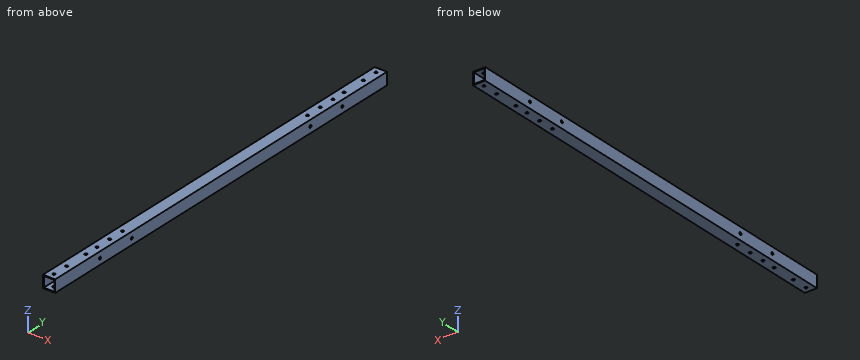
```python
from build123d import *

# Parameters (mm, degrees)
SKETCH_1_W          = 15
SKETCH_1_H          = 15
SKETCH_1_W_2        = 13
SKETCH_1_H_2        = 13
EXTRUDE_1_DEPTH     = 520
SKETCH_2_R          = 1.6
CUT_EXTRUDE_1_DEPTH = 521.270362408
SKETCH_3_R          = 1.6
CUT_EXTRUDE_2_DEPTH = 521.270362408


with BuildPart() as part:
    # 草图1 → 拉伸-薄壁1 (new body)
    with BuildSketch(Plane(origin=(0, 0, 0), x_dir=(1, 0, 0), z_dir=(0, 1, 0))):
        Rectangle(SKETCH_1_W, SKETCH_1_H)
        Rectangle(SKETCH_1_W_2, SKETCH_1_H_2, mode=Mode.SUBTRACT)
    extrude(amount=EXTRUDE_1_DEPTH)

    # 草图2 → 切除-拉伸1 (cut, through all)
    with BuildSketch(Plane.XY.offset(7.5)):
        with Locations((0, 7.5)):
            Circle(SKETCH_2_R)
        with Locations((0, 27.5)):
            Circle(SKETCH_2_R)
        with Locations((0, 57.5)):
            Circle(SKETCH_2_R)
        with Locations((0, 75)):
            Circle(SKETCH_2_R)
        with Locations((0, 95)):
            Circle(SKETCH_2_R)
        with Locations((0, 115)):
            Circle(SKETCH_2_R)
        with Locations(Location((0, 405, 0), (0, 0, 180))):
            Circle(SKETCH_2_R)
        with Locations(Location((0, 425, 0), (0, 0, 180))):
            Circle(SKETCH_2_R)
        with Locations(Location((0, 445, 0), (0, 0, 180))):
            Circle(SKETCH_2_R)
        with Locations(Location((0, 462.5, 0), (0, 0, 180))):
            Circle(SKETCH_2_R)
        with Locations(Location((0, 492.5, 0), (0, 0, 180))):
            Circle(SKETCH_2_R)
        with Locations(Location((0, 512.5, 0), (0, 0, 180))):
            Circle(SKETCH_2_R)
    extrude(amount=-CUT_EXTRUDE_1_DEPTH, mode=Mode.SUBTRACT)

    # 草图3 → 切除-拉伸2 (cut, through all)
    with BuildSketch(Plane(origin=(7.5, 0, 0), x_dir=(0, 0, -1), z_dir=(1, 0, 0))):
        with Locations((0, 70)):
            Circle(SKETCH_3_R)
        with Locations((0, 120)):
            Circle(SKETCH_3_R)
        with Locations((0, 400)):
            Circle(SKETCH_3_R)
        with Locations((0, 450)):
            Circle(SKETCH_3_R)
    extrude(amount=-CUT_EXTRUDE_2_DEPTH, mode=Mode.SUBTRACT)


solid = part.part
```
Verification items for the finished model (mm, model axes). Give positions to 0.01 mm unless a question says otherwise; leave off trailing zeros. Order: outer loops, then holes, each group sorted by start corner. A loop starts at its lowest first (then second) coordinate and runs counter-clockwise, first axis right, second up. Notation, with made-up numbers: M 22.5,-16 L 50.5,-16 A25 ccw 50.5,11 Z; hole C 6.5,12 d6. An arc over 180 degrees is marked long. Return JSON: item names as keys, results as strings. Group by question number.
1) Section check B-B on y = 274.5. Record the cut outline in (x, z), and give its area (3 significant figures).
2) Scan lines: line 1 (Z direction, x = -2, y = 469.5); line 2 (X direction, y = 492.5, z = -7.1). Record each from-to range of solid material in increasing order.
3) Section check A-A on x = 4. Record the cut outline in (y, z), and give its area (3 significant figures).
4) Go/stop test with flat-tipped pins: pin 1 Ø4 at (y, z) = (70, 0) entering from +X; pin 2 Ø1.5 at (x, z) = (-4, -0.5) entering from -Y. Record where each tip stops, or that it passes through.
Answer block:
{
 "1": {"outline": "M -7.5,-7.5 L 7.5,-7.5 L 7.5,7.5 L -7.5,7.5 Z; hole M -6.5,-6.5 L 6.5,-6.5 L 6.5,6.5 L -6.5,6.5 Z", "area": "56.0 mm^2"},
 "2": {"line 1": "z = -7.5 to -6.5, 6.5 to 7.5", "line 2": "x = -7.5 to -1.6, 1.6 to 7.5"},
 "3": {"outline": "M 0,-7.5 L 520,-7.5 L 520,-6.5 L 0,-6.5 Z; M 0,6.5 L 520,6.5 L 520,7.5 L 0,7.5 Z", "area": "1,040 mm^2"},
 "4": {"pin 1": "stops at x = 7.5", "pin 2": "passes through"}
}
